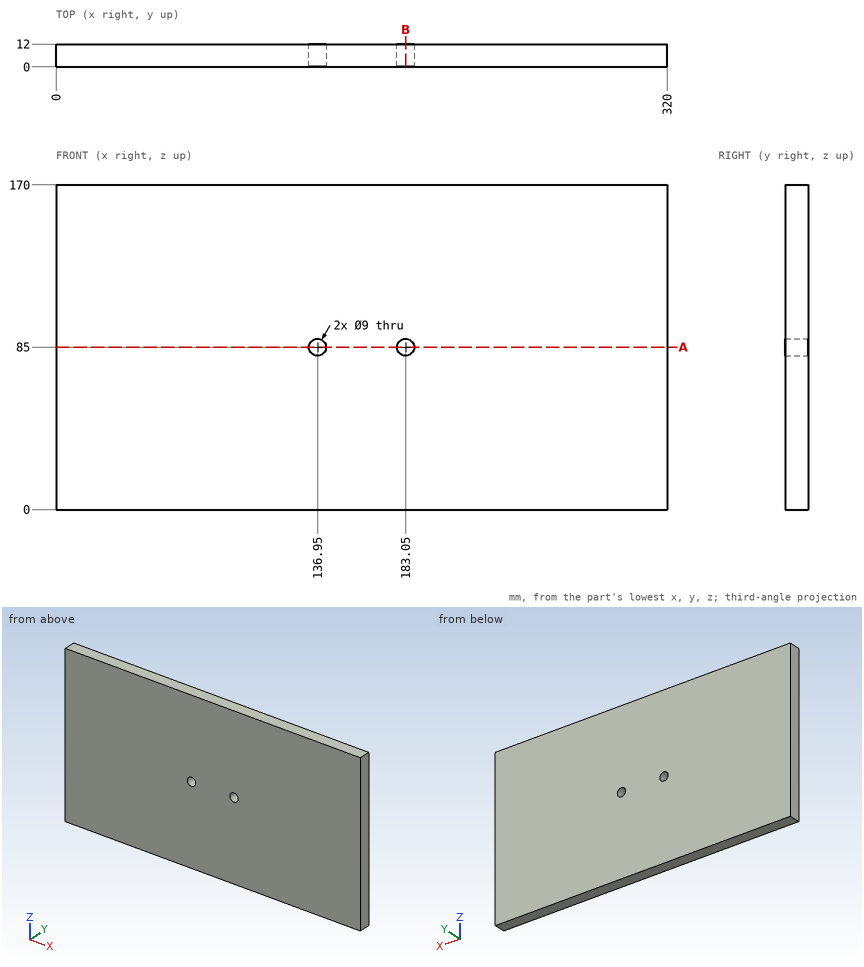
Here's the drawing with two shaded views (mm, measured from the low corner). I have some questions. Coordinates: 2 decimals unless noted, no trailing zeros. Write each loop counter-clockwise with the first axis right and the second up, starting at its lowest first coordinate (ties: lowest second). Pieces come first, ordered by that corner, then holes. Notation, with made-up numbers: (15.5, 43.5) -> (51.5, 43.5) arc R22 cw to (51.5, 73.5) -> close; hole circle Ø4 at (41, 45.25). An arc over 180 degrees is marked (long way). One line per question, with ' | ' between items. Start each with the question number.
1. If we section it at A-A (z = 85): Please give me the cut outline in (x, y), and give its area (3 significant figures).
2. If we section it at B-B (x = 183.05): Please give me the cut outline in (y, z), and give its area (3 significant figures).
3. Please list where these lines run through material, in increasing order: line 1 along X through (y, z) = (2.75, 85); line 2 along Z through (x, y) = (183.05, 5.25); line 3 along X through (y, z) = (2.5, 89).
Return value:
1) outline: (0, 0) -> (132.45, 0) -> (132.45, 12) -> (0, 12) -> close; (141.45, 0) -> (178.55, 0) -> (178.55, 12) -> (141.45, 12) -> close; (187.55, 0) -> (320, 0) -> (320, 12) -> (187.55, 12) -> close | area: 3,620 mm²
2) outline: (0, 0) -> (12, 0) -> (12, 80.5) -> (0, 80.5) -> close; (0, 89.5) -> (12, 89.5) -> (12, 170) -> (0, 170) -> close | area: 1,930 mm²
3) line 1: x = 0 to 132.45, 141.45 to 178.55, 187.55 to 320 | line 2: z = 0 to 80.5, 89.5 to 170 | line 3: x = 0 to 134.89, 139.01 to 180.99, 185.11 to 320
